Can you work these out from the model? Positions are in its coordinate system, mm. Face numbers are marked on the shaded views. A direction names the side the tool comes from. Give positions to 0.01 mm unless a question says otherwise; leave off trailing zeros. Loops run counter-clockwise (first coordinate to the right, second up) from the corner with the lowest first, then second, coordinate; pieces in that order, holes last. Notation, with made-up numbers: (-15, 49.25) - (34, 49.25) arc R31 cw to (34, 82.25) - close; hole circle Ø4 at (35, 32). An arc over 180 degrees is marked (long way). Answer as a JSON object with one key per item and string values. Group by question number.
Item 1: Will these pins go through, and if not, where does the flat tip stop? pin 1 (1 mm diameter, centred on x = 3, y = 1, fed in from -Z); pin 2 (2 mm diameter, centred on x = 4.5, z = -1.5, fed in from -Y).
Item 2: Suppose I cut it at B-B on x = 3. Write out the boundary of the cut face in (y, z), and give its area (3 significant figures).
Item 3: Please list where these lines run through material, in increasing order: L1, parallel to Y at x = 4.7, z = 0; L2, parallel to Y at x = 0.5, z = 1.75.
Item 4: Thinking about a two-plate mould opening in Z: for the marked faces 3, 4 and 5, which applies, pulls with the +Z half, pulls with the -Z half, needs draft (parallel to the pull), parting line crosses it, or undercut?
Item 5: Which directions (+Z, -Z, +X, -X, +Y, -Y) give clear straight access to the entire face, cutting with the end or side of a thin tool? Please do the marked faces 1 and 2.
Item 6: Suppose I cut it at A-A on x = 2.25. Write out the boundary of the cut face in (y, z).
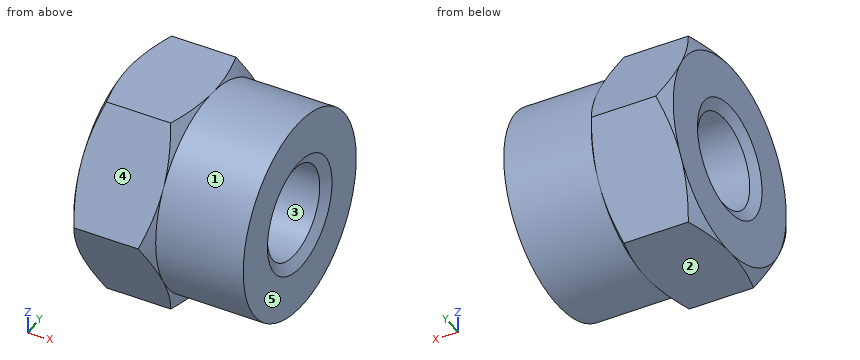
Autodesk Inventor part; units mm, degrees
ref_plane "Work Plane1" through (12.261, 0, 0) normal (0, 0, 1) x (-1, 0, 0)
ref_plane "YZ Plane" through (0, 0, 0) normal (1, 0, 0) x (0, 1, 0)
ref_plane "XZ Plane" through (0, 0, 0) normal (0, 1, 0) x (-1, 0, 0)
sketch "Sketch1" plane through (0, 0, 0) normal (1, 0, 0) x (0, 1, 0)
  line L0 (2.0207, -3.5) -> (-2.0207, -3.5)
  line L1 (-2.0207, -3.5) -> (-4.0415, 0)
  line L2 (-4.0415, 0) -> (-2.0207, 3.5)
  line L3 (-2.0207, 3.5) -> (2.0207, 3.5)
  line L4 (2.0207, 3.5) -> (4.0415, 0)
  line L5 (4.0415, 0) -> (2.0207, -3.5)
  point P0 (0, 0)
  point P1 (0, 0)
  dimension "d0" = 8.0829
extrude "Body" add sketch "Sketch1" along normal blind 2.9
sketch "Sketch2" plane through (2.9, 0, 0) normal (1, 0, 0) x (0, 0, -1)
  circle A0 centre (0, 0) radius 3.5
  dimension "d7" = 7
extrude "Ring" add sketch "Sketch2" along normal blind 3.1
sketch "Sketch3" plane through (0, 0, 0) normal (0, 0, 1) x (1, 0, 0)
  line L0 (0, 2.0207) -> (0, 4.0415)
  line L1 (0, 4.0415) -> (2.9, 4.0415)
  line L2 (2.9, 2.0207) -> (2.9, 4.0415)
  line L3 (-0.58, 0) -> (3.48, 0)
  line L4 (0, 3.5) -> (0.3126, 4.0415)
  line L5 (2.5874, 4.0415) -> (2.9, 3.5)
  dimension "d3" = 30
  dimension "d4" = 30
  dimension "d5" = 7
  dimension "d6" = 7
revolve "Chamfer1" cut sketch "Sketch3" angle 360 about axis through (-10, 0, 0) along (1, 0, 0)
sketch "Sketch4" plane through (0, 0, 0) normal (-1, 0, 0) x (0, 0, 1)
  line L0 (0, -5.658) -> (0, 5.658)
  line L1 (-4.9, 0) -> (4.9, 0)
  point P0 (0, 0)
hole "Thread" at (0, 0, 0) direction (1, 0, 0) diameter 3.242 end through all
chamfer "Chamfer2" distance 0.3789 angle 30 1 edges at (0, 0, -1.621) measured on face at (0, 2.8569, 0.0651)
chamfer "Chamfer3" distance 0.3789 angle 30 1 edges at (6, 0, -1.621) measured on face at (6, -0.4085, -2.8241)
ref_plane "Work Plane1" through (12.261, 0, 0) normal (0, 0, 1) x (-1, 0, 0)
equation "\"d0\" = 1.1547 * SW"
equation "\"d1\" = KOH1"
equation "\"d7\" = SD2"
equation "\"d8\" = KOH - KOH1"
equation "\"d3\" = ANG1"
equation "\"d4\" = ANG2"
equation "\"d5\" = SW0"
equation "\"d6\" = SW01"
equation "\"d10\" = -0.5 * GD1 + 0.5 * NND"
equation "\"d46\" = -0.5 * GD1 + 0.5 * NND"
equation "\"d12\" = -0.5 * GD1 + 0.5 * NND"
equation "\"d47\" = -0.5 * GD1 + 0.5 * NND"
equation "\"ANG1\" = 30deg"
equation "\"ANG2\" = ANG1"
equation "\"NND\" = 4"
equation "\"KOH1\" = 2.9"
equation "\"KOH\" = 6"
equation "\"SW\" = 7"
equation "\"SW0\" = SW"
equation "\"SW01\" = SW"
equation "\"SD2\" = SW"
equation "\"GUL\" = 0.541266 * PTC"
equation "\"THREADDIA\" = 4"
equation "\"TOA\" = 30deg"
equation "\"PTC\" = 0.7"
equation "\"E0\" = 1.155 * SW"
equation "\"GAL\" = 0.541266 * PTC"
properties part number "NF E 25-409 - M4" material "Steel, Mild"
Worked out:
{
 "1": {"pin 1": "stops at z = -3.5", "pin 2": "stops at y = -3.46"},
 "2": {"outline": "circle Ø7 at (0, 0); hole circle Ø3.24 at (0, 0)", "area": "30.2 mm2"},
 "3": {"L1": "y = -3.5 to -1.62, 1.62 to 3.5", "L2": "y = -3.03 to 3.03"},
 "4": {"face 3": "undercut", "face 4": "pulls with the +Z half", "face 5": "needs draft"},
 "5": {"face 1": "+X", "face 2": "-Z, +X, -X, +Y, -Y"},
 "6": {"outline": "(-4.04, 0) - (-2.02, -3.5) - (2.02, -3.5) - (4.04, 0) - (2.02, 3.5) - (-2.02, 3.5) - close; hole circle Ø3.24 at (0, 0)"}
}
